Check sheet for the drawn part. Datum: minimum x, y, z corner. Units: mm. Round coordinates to 2 decimals unless told otherwise and drop trailing zeros. Write each loop counter-clockwise with the first axis right and the second up, starting at its lowest first coordinate (ties: lowest second). Pieces come first, ordered by that corner, then holes. Notation, with made-up numbers: M -28.5,34 L 9.5,34 A16 cw 9.5,46 Z; hole C 11,-13 d9. An arc over 180 degrees is marked long. One line per item, written item: value.
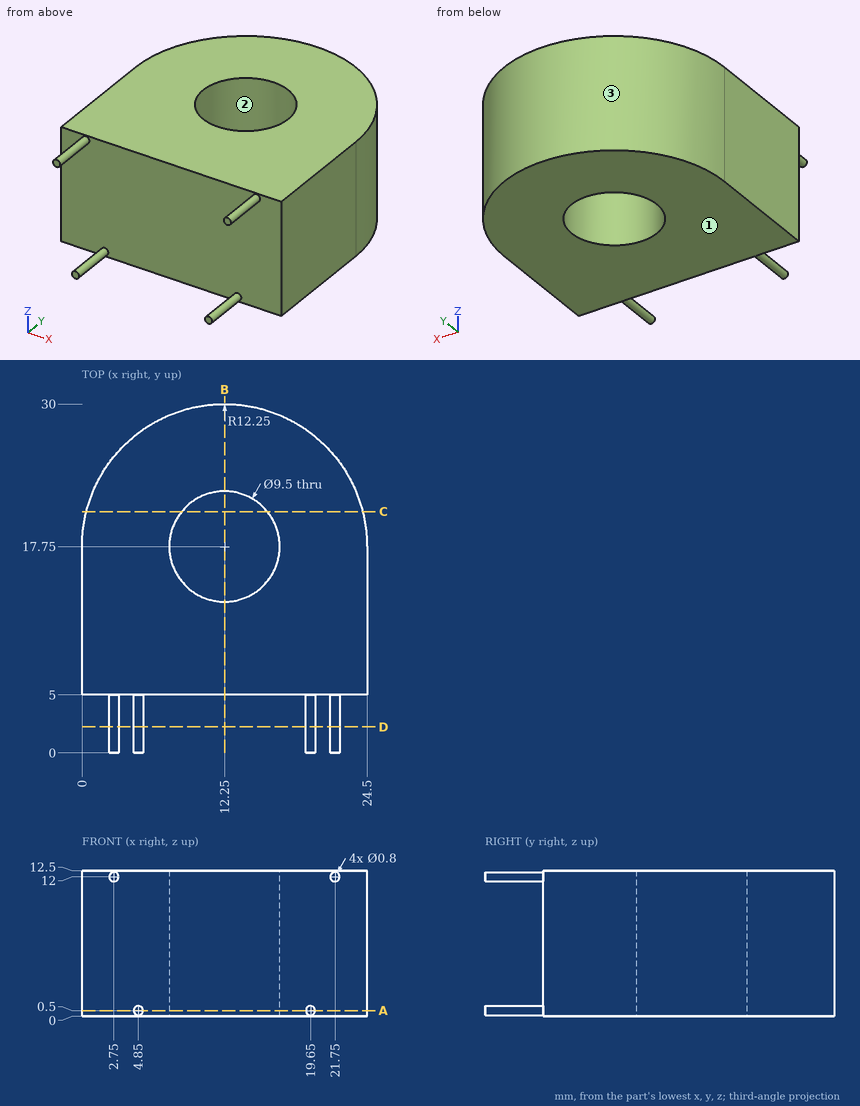
Q1. Sectioned sample at C-C on y = 20.75. Enter the section's corners in (x, z).
Completed:
outline: M 0.37,0 L 8.57,0 L 8.57,12.5 L 0.37,12.5 Z; M 15.93,0 L 24.13,0 L 24.13,12.5 L 15.93,12.5 Z
Q2. Draft check along Y on the marked faces 1, 2 and 3. Enter one of: pulls with the +Y half, pulls with the -Y half, needs draft (parallel to the pull), parting line crosses it, or undercut.
Completed:
face 1: needs draft
face 2: undercut
face 3: pulls with the +Y half
Q3. Sectioned sample at A-A on z = 0.5. Enter the section's corners in (x, y), and give its area (3 significant figures).
Completed:
outline: M 0,5 L 4.45,5 L 4.45,0 L 5.25,0 L 5.25,5 L 19.25,5 L 19.25,0 L 20.05,0 L 20.05,5 L 24.5,5 L 24.5,17.75 A12.25 ccw 0,17.75 Z; hole C 12.25,17.75 d9.5
area: 485 mm^2
Q4. Scan lines: line 1 (Y direction, x = 12.25, z = 8); line 2 (Y direction, x = 15, z = 5.25); line 3 (X direction, y = 17.5, z = 6.25). Record each from-to range of solid material in increasing order. Write a range as [from, to].
Completed:
line 1: [5, 13], [22.5, 30]
line 2: [5, 13.88], [21.62, 29.69]
line 3: [0, 7.51], [16.99, 24.5]
Q5. Sectioned sample at B-B on x = 12.25. Enter the section's corners in (y, z).
Completed:
outline: M 5,0 L 13,0 L 13,12.5 L 5,12.5 Z; M 22.5,0 L 30,0 L 30,12.5 L 22.5,12.5 Z
Q6. Sectioned sample at D-D on y = 2.25. Enter the section's corners in (x, z), and give its area (3 significant figures).
Completed:
outline: C 2.75,12 d0.8; C 4.85,0.5 d0.8; C 19.65,0.5 d0.8; C 21.75,12 d0.8
area: 2.01 mm^2
